from build123d import *

# Parameters (mm, degrees)
SKETCH1_W           = 76.2
SKETCH1_H           = 76.2
SKETCH1_R           = 3.229097739
BOSS_EXTRUDE3_DEPTH = 3.175
CUT_EXTRUDE1_DEPTH  = 3.175


with BuildPart() as part:
    # Sketch1 → Boss-Extrude3 (new body)
    with BuildSketch(Plane.XY):
        with Locations((38.1, 38.1)):
            Rectangle(SKETCH1_W, SKETCH1_H)
        with Locations((6.35, 69.596)):
            Circle(SKETCH1_R, mode=Mode.SUBTRACT)
        with Locations((6.35, 6.604)):
            Circle(SKETCH1_R, mode=Mode.SUBTRACT)
        with Locations((65.2018, 67.945)):
            Circle(SKETCH1_R, mode=Mode.SUBTRACT)
        with Locations((65.2018, 8.255)):
            Circle(SKETCH1_R, mode=Mode.SUBTRACT)
    extrude(amount=BOSS_EXTRUDE3_DEPTH)

    # Sketch2 → Cut-Extrude1 (cut)
    with BuildSketch(Plane.XY.offset(3.175)):
        with BuildLine():
            Line((15.875, 44.45), (60.325, 44.45))
            ThreePointArc((60.325, 44.45), (66.675, 38.1), (60.325, 31.75))
            Line((60.325, 31.75), (15.875, 31.75))
            ThreePointArc((15.875, 31.75), (9.525, 38.1), (15.875, 44.45))
        make_face()
    extrude(amount=-CUT_EXTRUDE1_DEPTH, mode=Mode.SUBTRACT)


solid = part.part
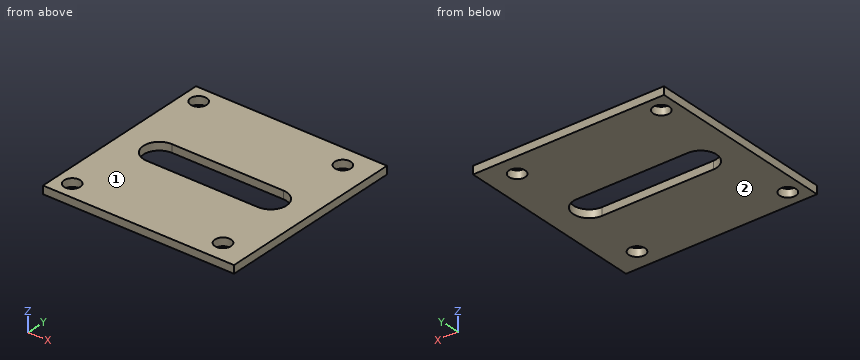
Geometry: final body of the model. Coordinates: model frame, mm. Face numbers are marked on the shaded views. Coordinates: 2 decimals unless noted, no trailing zeros. Write each loop counter-clockwise with the first axis right and the second up, starting at its lowest first coordinate (ties: lowest second). Pieces come first, ordered by that corner, then holes. Notation, with made-up numbers: (29, 16.25) - (45, 16.25) arc R12 cw to (45, 37.25) - close; hole circle Ø6 at (18.5, -37). An arc over 180 degrees is marked (long way). Return JSON: item names as keys, results as strings.
Item 1: Section query A-A (x = 49). Output: boundary loops of the cut face in (y, z) (3 decimals).
Completed:
{"outline": "(0, 0) - (31.75, 0) - (31.75, 3.175) - (0, 3.175) - close; (44.45, 0) - (76.2, 0) - (76.2, 3.175) - (44.45, 3.175) - close"}
Item 2: Section query D-D (z = 2.15). Output: boundary loops of the cut face in (x, y) (3 decimals), and give its area (3 significant figures).
Completed:
{"outline": "(0, 0) - (76.2, 0) - (76.2, 76.2) - (0, 76.2) - close; hole circle Ø6.458 at (6.35, 6.604); hole circle Ø6.458 at (6.35, 69.596); hole (15.875, 31.75) - (60.325, 31.75) arc R6.35 ccw to (60.325, 44.45) - (15.875, 44.45) arc R6.35 ccw to start; hole circle Ø6.458 at (65.202, 8.255); hole circle Ø6.458 at (65.202, 67.945)", "area": "4,980 mm2"}
Item 3: Section query C-C (x = 6.35). Output: boundary loops of the cut face in (y, z) (3 decimals).
Completed:
{"outline": "(0, 0) - (3.375, 0) - (3.375, 3.175) - (0, 3.175) - close; (9.833, 0) - (66.367, 0) - (66.367, 3.175) - (9.833, 3.175) - close; (72.825, 0) - (76.2, 0) - (76.2, 3.175) - (72.825, 3.175) - close"}
Item 4: Pull-direction query (Z, two-part tool) for the marked faces 1 and 2; classes: +Z half, -Z half, draft (parallel to the pull), parting line (faces both ways), or undercut.
Completed:
{"face 1": "+Z half", "face 2": "-Z half"}
Item 5: Section query B-B (y = 38.1). Output: boundary loops of the cut face in (x, z) (3 decimals).
Completed:
{"outline": "(0, 0) - (9.525, 0) - (9.525, 3.175) - (0, 3.175) - close; (66.675, 0) - (76.2, 0) - (76.2, 3.175) - (66.675, 3.175) - close"}
Item 6: Line query: L1, parallel to Y at x = 6.35, z = 2.1; L2, parallel to Y at x = 32.5, z = 0.45; L3, parallel to Y at x = 64.5, z = 3. Output: solid intervals per line, ascending.
Completed:
{"L1": "y = 0 to 3.37, 9.83 to 66.37, 72.83 to 76.2", "L2": "y = 0 to 31.75, 44.45 to 76.2", "L3": "y = 0 to 5.1, 11.41 to 33.32, 42.88 to 64.79, 71.1 to 76.2"}
